Design review of the part built by this model. Coordinates are the model's own, in mm. A direction names the side the tool comes from. Coordinates: 2 decimals unless noted, no trailing zeros. Write each loop counter-clockwise with the first axis right and the second up, starting at its lowest first coordinate (ties: lowest second). Pieces come first, ordered by that corner, then holes. Notation, with made-up numbers: (-9, 26) - (37, 26) arc R21 cw to (37, 65) - close; hole circle Ø3 at (-37, 79). An arc over 180 degrees is marked (long way). Use a Markdown table: item, result.
from build123d import *

# Parameters (mm, degrees)
ESQUISSE1_W             = 32
ESQUISSE1_H             = 19
BOSS_EXTRU_1_DEPTH      = 9
ESQUISSE2_R             = 5.5
ESQUISSE2_R_2           = 1.25
ESQUISSE2_R_3           = 1.65
ENL_V_MAT_EXTRU_1_DEPTH = 39.288379438
ESQUISSE3_W             = 2
ESQUISSE3_H             = 7
ENL_V_MAT_EXTRU_2_DEPTH = 39.288379438
ESQUISSE4_W             = 28
ESQUISSE4_H             = 2
BOSS_EXTRU_2_DEPTH      = 9
CHANFREIN1_SIZE         = 5


with BuildPart() as part:
    # Esquisse1 → Boss.-Extru.1 (new body)
    with BuildSketch(Plane.XY):
        with Locations((16, 9.5)):
            Rectangle(ESQUISSE1_W, ESQUISSE1_H)
    extrude(amount=BOSS_EXTRU_1_DEPTH)

    # Esquisse2 → Enlèv. mat.-Extru.1 (cut, through all)
    with BuildSketch(Plane.XY.offset(9)):
        with Locations((16, 12)):
            Circle(ESQUISSE2_R)
        with Locations((8.221825407, 12)):
            Circle(ESQUISSE2_R_2)
        with Locations(Location((23.778174593, 12, 0), (0, 0, 180))):
            Circle(ESQUISSE2_R_2)
        with Locations((16, 4.221825407)):
            Circle(ESQUISSE2_R_2)
        with Locations((5, 3)):
            Circle(ESQUISSE2_R_3)
        with Locations(Location((27, 3, 0), (0, 0, 180))):
            Circle(ESQUISSE2_R_3)
    extrude(amount=-ENL_V_MAT_EXTRU_1_DEPTH, mode=Mode.SUBTRACT)

    # Esquisse3 → Enlèv. mat.-Extru.2 (cut, through all)
    with BuildSketch(Plane.XY.offset(9)):
        with Locations((1, 3.5)):
            Rectangle(ESQUISSE3_W, ESQUISSE3_H)
        with Locations((31, 3.5)):
            Rectangle(ESQUISSE3_W, ESQUISSE3_H)
    extrude(amount=-ENL_V_MAT_EXTRU_2_DEPTH, mode=Mode.SUBTRACT)

    # Esquisse4 → Boss.-Extru.2 (add)
    with BuildSketch(Plane.XY.offset(9)):
        with Locations((16, -1)):
            Rectangle(ESQUISSE4_W, ESQUISSE4_H)
    extrude(amount=-BOSS_EXTRU_2_DEPTH)

    # Chanfrein1
    chanfrein1_edges = [part.edges().sort_by_distance(p)[0] for p in [
        (0, 19, 4.5),
        (32, 19, 4.5),
    ]]
    chamfer(chanfrein1_edges, length=CHANFREIN1_SIZE)


solid = part.part
(1) Take a section at D-D on x = 11.5. Write out the cut boundary in (y, z), and give its area (3 significant figures).
Determined:
| item | result |
|---|---|
| outline | (-2, 0) - (8.84, 0) - (8.84, 9) - (-2, 9) - close; (15.16, 0) - (19, 0) - (19, 9) - (15.16, 9) - close |
| area | 132 mm2 |
(2) For pin 1 (1.5 mm diameter, centred on x = 8.5, y = 9.5, fed in from -Z); pin 2 (4.5 mm diameter, centred on y = 4.5, z = 4.5, fed in from +X); pin 3 (0.6 mm diameter, centred on x = 31, z = 2.5, fed in from -Y); pin 4 (1.5 mm diameter, centred on x = 4, z = 5, fed in from +Y), all flat-tipped, find the tip position at first contact; note any pin that passes through.
Determined:
| item | result |
|---|---|
| pin 1 | z = 0 |
| pin 2 | x = 30 |
| pin 3 | y = 7 |
| pin 4 | y = 18.75 |
(3) Machinability: for faces 1 (the flat face through (1, 7, 5)), 2 (the flat face through (16, 19, 4)), 3 (the flat face through (30, 2, 5)), which of the approach directions +Z, -Z, +X, -X, +Y, -Y give a long, thin tool a straight path to every point of the face, cutting with its end or side? Answer none if there is none.
Determined:
| item | result |
|---|---|
| face 1 | +Z, -Z, -X, -Y |
| face 2 | +Z, -Z, +X, -X, +Y |
| face 3 | +Z, -Z, +X, -Y |
(4) Take a section at A-A on x = 16. Write out the cut boundary in (y, z), and give its area (3 significant figures).
Determined:
| item | result |
|---|---|
| outline | (-2, 0) - (2.97, 0) - (2.97, 9) - (-2, 9) - close; (5.47, 0) - (6.5, 0) - (6.5, 9) - (5.47, 9) - close; (17.5, 0) - (19, 0) - (19, 9) - (17.5, 9) - close |
| area | 67.5 mm2 |
(5) Draft analysis for pull direction X (two halves, no side actions). For faces 4 (the flat face through (2, 2, 5)), 5 (the flat face through (16, 6, 9)), 6 (the cylindrical face through (8.06, 13.24, 4.56)), state which applies: +X half, -X half, draft (parallel to the pull), parting line (faces both ways), or undercut.
Determined:
| item | result |
|---|---|
| face 4 | -X half |
| face 5 | draft |
| face 6 | undercut |
(6) Take a section at B-B on y = 16.5. Write out the cut boundary in (x, z).
Determined:
| item | result |
|---|---|
| outline | (2.5, 0) - (12.84, 0) - (12.84, 9) - (2.5, 9) - close; (19.16, 0) - (29.5, 0) - (29.5, 9) - (19.16, 9) - close |
(7) Take a section at C-C on z = 4.75. Write out the cut boundary in (x, y).
Determined:
| item | result |
|---|---|
| outline | (0, 7) - (2, 7) - (2, -2) - (30, -2) - (30, 7) - (32, 7) - (32, 14) - (27, 19) - (5, 19) - (0, 14) - close; hole circle Ø3.3 at (5, 3); hole circle Ø2.5 at (8.22, 12); hole circle Ø11 at (16, 12); hole circle Ø2.5 at (16, 4.22); hole circle Ø2.5 at (23.78, 12); hole circle Ø3.3 at (27, 3) |
(8) For L1, parallel to Y at x = 16, z = 4.5; L2, parallel to X at y = 12.5, z = 8; L3, parallel to Y at x = 15, z = 4.75, list the stretches that pass through material, from the lowest coordinate up. Write a range as from..to.
Determined:
| item | result |
|---|---|
| L1 | -2..2.97, 5.47..6.5, 17.5..19 |
| L2 | 0..7.08, 9.37..10.52, 21.48..22.63, 24.92..32 |
| L3 | -2..3.47, 4.97..6.59, 17.41..19 |
